from build123d import *

# Parameters (mm, degrees)
F0_R     = 2.38125
F1_DEPTH = 3.175


with BuildPart() as f1:
    # F0 (on Right) → F1 (new body)
    with BuildSketch(Plane.YZ):
        with BuildLine():
            Line((505.190684, 4.7625), (0, 4.7625))
            ThreePointArc((0, 4.7625), (-4.7625, 0), (0, -4.7625))
            Line((0, -4.7625), (505.190684, -4.7625))
            ThreePointArc((505.190684, -4.7625), (509.953184, 0), (505.190684, 4.7625))
        make_face()
        Circle(F0_R, mode=Mode.SUBTRACT)
        with Locations((252.595342, 0)):
            Circle(F0_R, mode=Mode.SUBTRACT)
        with Locations((505.190684, 0)):
            Circle(F0_R, mode=Mode.SUBTRACT)
    extrude(amount=F1_DEPTH)


solid = f1.part
Geometry check sheet. Reference: the model listing, model coordinates, mm. Give positions to 0.01 mm unless a question says otherwise; leave off trailing zeros. Order: outer loops, then holes, each group sorted by start corner. A loop starts at its lowest first (then second) coordinate and runs counter-clockwise, first axis right, second up. Notation, with made-up numbers: (-22.5, 3.25) - (4.5, 3.25) arc R16 cw to (4.5, 16.25) - close; hole circle Ø7 at (44, 61). An arc over 180 degrees is marked (long way). Answer as a JSON object with one key per item and string values.
(1) Cross-section at A-A (z = 0). Record the cut outline in (x, y) (1 decimal).
Report:
{"outline": "(0, -4.8) - (3.2, -4.8) - (3.2, -2.4) - (0, -2.4) - close; (0, 2.4) - (3.2, 2.4) - (3.2, 250.2) - (0, 250.2) - close; (0, 255) - (3.2, 255) - (3.2, 502.8) - (0, 502.8) - close; (0, 507.6) - (3.2, 507.6) - (3.2, 510) - (0, 510) - close"}
(2) Material ranges on line 1 (Y direction, x = 1.35, z = -0.75); line 2 (Y direction, x = 2.45, z = 1.25); line 3 (Y direction, x = 0.3, z = 2.5), recorded low to high.
Report:
{"line 1": "-4.7 to -2.26, 2.26 to 250.34, 254.86 to 502.93, 507.45 to 509.89", "line 2": "-4.6 to -2.03, 2.03 to 250.57, 254.62 to 503.16, 507.22 to 509.79", "line 3": "-4.05 to 509.24"}
(3) Depth check by flat-ended pin: pin 1 Ø4 at (y, z) = (252.6, 0) entering from -X (3 decimals). Enter the tip coordinate at first touch or a pass-through.
Report:
{"pin 1": "through"}
